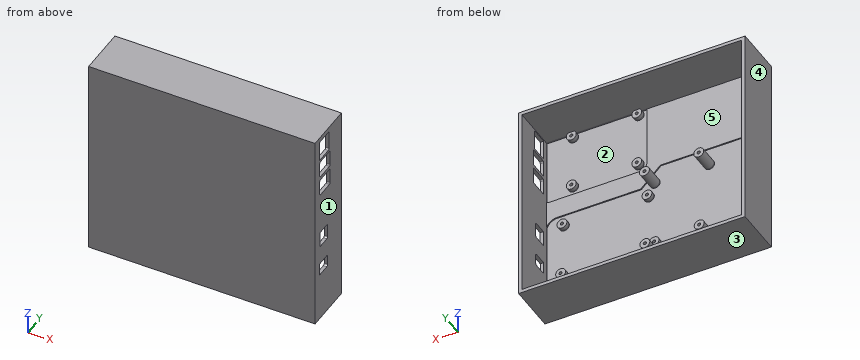
from build123d import *

# Parameters (mm, degrees)
SKETCH1_W           = 200.4
SKETCH1_H           = 180.383316975
SKETCH1_W_2         = 194.4
SKETCH1_H_2         = 174.383316975
BOSS_EXTRUDE1_DEPTH = 3
SKETCH1_3_W         = 200.4
SKETCH1_3_H         = 180.383316975
SKETCH1_3_W_2       = 194.4
SKETCH1_3_H_2       = 174.383316975
BOSS_EXTRUDE2_DEPTH = 40
SKETCH2_R           = 4.4
SKETCH2_R_2         = 1.4
BOSS_EXTRUDE3_DEPTH = 3
BOSS_EXTRUDE4_START = 3
SKETCH2_2_R         = 4.4
SKETCH2_2_R_2       = 1.4
BOSS_EXTRUDE4_DEPTH = 13.67
SKETCH3_R           = 4.4
CUT_EXTRUDE1_DEPTH  = 1
CUT_EXTRUDE2_DEPTH  = 5


with BuildPart() as part:
    # Sketch1 → Boss-Extrude1 (new body)
    with BuildSketch(Plane(origin=(0, -4, 0), x_dir=(-1, 0, 0), z_dir=(0, -1, 0))):
        with Locations((47.125, -25.608341513)):
            Rectangle(SKETCH1_W, SKETCH1_H)
        with Locations((47.125, -25.608341513)):
            Rectangle(SKETCH1_W_2, SKETCH1_H_2, mode=Mode.SUBTRACT)
        with Locations((47.125, -25.608341513)):
            Rectangle(SKETCH1_W_2, SKETCH1_H_2)
    extrude(amount=BOSS_EXTRUDE1_DEPTH)

    # Sketch1<3> → Boss-Extrude2 (add)
    with BuildSketch(Plane(origin=(0, -4, 0), x_dir=(-1, 0, 0), z_dir=(0, -1, 0))):
        with Locations((47.125, -25.608341513)):
            Rectangle(SKETCH1_3_W, SKETCH1_3_H)
        with Locations((47.125, -25.608341513)):
            Rectangle(SKETCH1_3_W_2, SKETCH1_3_H_2, mode=Mode.SUBTRACT)
    extrude(amount=-BOSS_EXTRUDE2_DEPTH)

    # Sketch2 → Boss-Extrude3 (add)
    with BuildSketch(Plane(origin=(0, -4, 0), x_dir=(1, 0, 0), z_dir=(0, 1, 0))):
        with Locations(Location((-94.083642028, 35.599553337, 0), (0, 0, 90))):
            Circle(SKETCH2_R)
        with Locations(Location((-94.083642028, 35.599553337, 0), (0, 0, 270))):
            Circle(SKETCH2_R_2, mode=Mode.SUBTRACT)
        with Locations(Location((-45.977533902, 35.843746779, 0), (0, 0, 90))):
            Circle(SKETCH2_R)
        with Locations(Location((-45.977533902, 35.843746779, 0), (0, 0, 270))):
            Circle(SKETCH2_R_2, mode=Mode.SUBTRACT)
        with Locations(Location((-46.675, 24.55, 0), (0, 0, 90))):
            Circle(SKETCH2_R)
        with Locations(Location((-46.675, 24.55, 0), (0, 0, 270))):
            Circle(SKETCH2_R_2, mode=Mode.SUBTRACT)
        with Locations(Location((35.975, 24.55, 0), (0, 0, 90))):
            Circle(SKETCH2_R)
        with Locations(Location((35.975, 24.55, 0), (0, 0, 270))):
            Circle(SKETCH2_R_2, mode=Mode.SUBTRACT)
        with Locations(Location((-40.425, -24.5, 0), (0, 0, 90))):
            Circle(SKETCH2_R)
        with Locations(Location((-40.425, -24.5, 0), (0, 0, 270))):
            Circle(SKETCH2_R_2, mode=Mode.SUBTRACT)
        with Locations(Location((-93.717351865, -36.559608852, 0), (0, 0, 90))):
            Circle(SKETCH2_R)
        with Locations(Location((-93.717351865, -36.559608852, 0), (0, 0, 270))):
            Circle(SKETCH2_R_2, mode=Mode.SUBTRACT)
        with Locations(Location((-45.611243739, -36.31541541, 0), (0, 0, 90))):
            Circle(SKETCH2_R)
        with Locations(Location((-45.611243739, -36.31541541, 0), (0, 0, 270))):
            Circle(SKETCH2_R_2, mode=Mode.SUBTRACT)
        with Locations(Location((34.775, -24.5, 0), (0, 0, 90))):
            Circle(SKETCH2_R)
        with Locations(Location((34.775, -24.5, 0), (0, 0, 270))):
            Circle(SKETCH2_R_2, mode=Mode.SUBTRACT)
        with Locations(Location((-31.425, -60.3, 0), (0, 0, 90))):
            Circle(SKETCH2_R)
        with Locations(Location((-31.425, -60.3, 0), (0, 0, 270))):
            Circle(SKETCH2_R_2, mode=Mode.SUBTRACT)
        with Locations(Location((26.575, -60.3, 0), (0, 0, 90))):
            Circle(SKETCH2_R)
        with Locations(Location((26.575, -60.3, 0), (0, 0, 270))):
            Circle(SKETCH2_R_2, mode=Mode.SUBTRACT)
        with Locations((-31.425, -109.3)):
            Circle(SKETCH2_R)
        with Locations(Location((-31.425, -109.3, 0), (0, 0, 270))):
            Circle(SKETCH2_R_2, mode=Mode.SUBTRACT)
        with Locations((26.575, -109.3)):
            Circle(SKETCH2_R)
        with Locations(Location((26.575, -109.3, 0), (0, 0, 270))):
            Circle(SKETCH2_R_2, mode=Mode.SUBTRACT)
    extrude(amount=BOSS_EXTRUDE3_DEPTH)

    # Sketch2<2> → Boss-Extrude4 (add)
    with BuildSketch(Plane(origin=(0, -4, 0), x_dir=(1, 0, 0), z_dir=(0, 1, 0)).offset(BOSS_EXTRUDE4_START)):
        with Locations(Location((-93.717351865, -36.559608852, 0), (0, 0, 90))):
            Circle(SKETCH2_2_R)
        with Locations(Location((-93.717351865, -36.559608852, 0), (0, 0, 270))):
            Circle(SKETCH2_2_R_2, mode=Mode.SUBTRACT)
        with Locations(Location((-45.611243739, -36.31541541, 0), (0, 0, 90))):
            Circle(SKETCH2_2_R)
        with Locations(Location((-45.611243739, -36.31541541, 0), (0, 0, 270))):
            Circle(SKETCH2_2_R_2, mode=Mode.SUBTRACT)
        with Locations(Location((-45.977533902, 35.843746779, 0), (0, 0, 90))):
            Circle(SKETCH2_2_R)
        with Locations(Location((-45.977533902, 35.843746779, 0), (0, 0, 270))):
            Circle(SKETCH2_2_R_2, mode=Mode.SUBTRACT)
        with Locations(Location((-94.083642028, 35.599553337, 0), (0, 0, 90))):
            Circle(SKETCH2_2_R)
        with Locations(Location((-94.083642028, 35.599553337, 0), (0, 0, 270))):
            Circle(SKETCH2_2_R_2, mode=Mode.SUBTRACT)
    extrude(amount=BOSS_EXTRUDE4_DEPTH)

    # Sketch3 → Cut-Extrude1 (cut)
    with BuildSketch(Plane(origin=(0, -4, 0), x_dir=(1, 0, 0), z_dir=(0, 1, 0))):
        with BuildLine():
            ThreePointArc((-133.325, -42.184637589), (-130.587997755, -49.351043774), (-123.472052941, -52.216683025))
            Line((-123.472052941, -52.216683025), (-50.730015352, -52.216683025))
            Line((-50.730015352, -52.216683025), (-33.377368591, -35.013077971))
            Line((-33.377368591, -35.013077971), (40.937843176, -35.013077971))
            ThreePointArc((40.937843176, -35.013077971), (46.610387698, -33.142667164), (50.075, -28.277211426))
            Line((50.075, -28.277211426), (50.075, 27.447920543))
            ThreePointArc((50.075, 27.447920543), (46.449358415, 32.437948869), (40.534398357, 34.186922029))
            Line((40.534398357, 34.186922029), (-33.678452679, 34.186922029))
            Line((-33.678452679, 34.186922029), (-50.108918246, 50.583316975))
            Line((-50.108918246, 50.583316975), (-124.102104511, 50.583316975))
            ThreePointArc((-124.102104511, 50.583316975), (-130.528855148, 47.775760881), (-133.325, 41.344037245))
            Line((-133.325, 41.344037245), (-133.325, -42.184637589))
        make_face()
        with Locations(Location((-93.717351865, -36.559608852, 0), (0, 0, 270))):
            Circle(SKETCH3_R, mode=Mode.SUBTRACT)
        with Locations(Location((-45.611243739, -36.31541541, 0), (0, 0, 270))):
            Circle(SKETCH3_R, mode=Mode.SUBTRACT)
        with Locations(Location((-94.083642028, 35.599553337, 0), (0, 0, 270))):
            Circle(SKETCH3_R, mode=Mode.SUBTRACT)
        with Locations(Location((-40.425, -24.5, 0), (0, 0, 270))):
            Circle(SKETCH3_R, mode=Mode.SUBTRACT)
        with Locations(Location((34.775, -24.5, 0), (0, 0, 270))):
            Circle(SKETCH3_R, mode=Mode.SUBTRACT)
        with Locations(Location((-46.675, 24.55, 0), (0, 0, 270))):
            Circle(SKETCH3_R, mode=Mode.SUBTRACT)
        with Locations(Location((-45.977533902, 35.843746779, 0), (0, 0, 270))):
            Circle(SKETCH3_R, mode=Mode.SUBTRACT)
        with Locations(Location((35.975, 24.55, 0), (0, 0, 270))):
            Circle(SKETCH3_R, mode=Mode.SUBTRACT)
        with BuildLine():
            Line((50.075, -112.8), (50.075, -53.47544468))
            ThreePointArc((50.075, -53.47544468), (48.612548822, -52.970948556), (47.075, -52.8))
            Line((47.075, -52.8), (-31.925, -52.8))
            ThreePointArc((-31.925, -52.8), (-36.874747468, -54.850252532), (-38.925, -59.8))
            Line((-38.925, -59.8), (-38.925, -109.8))
            ThreePointArc((-38.925, -109.8), (-38.754051444, -111.337548822), (-38.24955532, -112.8))
            Line((-38.24955532, -112.8), (-34.091458325, -112.8))
            ThreePointArc((-34.091458325, -112.8), (-31.425, -104.9), (-28.758541675, -112.8))
            Line((-28.758541675, -112.8), (23.908541675, -112.8))
            ThreePointArc((23.908541675, -112.8), (26.575, -104.9), (29.241458325, -112.8))
            Line((29.241458325, -112.8), (50.075, -112.8))
        make_face()
        with Locations(Location((-31.425, -60.3, 0), (0, 0, 270))):
            Circle(SKETCH3_R, mode=Mode.SUBTRACT)
        with Locations(Location((26.575, -60.3, 0), (0, 0, 270))):
            Circle(SKETCH3_R, mode=Mode.SUBTRACT)
    extrude(amount=-CUT_EXTRUDE1_DEPTH, mode=Mode.SUBTRACT)

    # Sketch4 → Cut-Extrude2 (cut)
    with BuildSketch(Plane(origin=(53.075, 0, 0), x_dir=(0, 0, -1), z_dir=(1, 0, 0))):
        with BuildLine():
            Line((9.9, 0.63), (20.9, 0.63))
            Line((20.9, 0.63), (20.9, 12.13))
            ThreePointArc((20.9, 12.13), (20.460660172, 13.190660172), (19.4, 13.63))
            Line((19.4, 13.63), (11.4, 13.63))
            ThreePointArc((11.4, 13.63), (10.339339828, 13.190660172), (9.9, 12.13))
            Line((9.9, 12.13), (9.9, 0.63))
        make_face()
        with BuildLine():
            Line((-8.32, 13.68), (-19.44, 13.68))
            ThreePointArc((-19.44, 13.68), (-20.472375901, 13.252375901), (-20.9, 12.22))
            Line((-20.9, 12.22), (-20.9, 12.12))
            Line((-20.9, 12.12), (-20.9, 2.47))
            Line((-20.9, 2.47), (-20.9, 1.06))
            Line((-20.9, 1.06), (-6.86, 1.06))
            Line((-6.86, 1.06), (-6.86, 2.47))
            Line((-6.86, 2.47), (-6.86, 12.12))
            Line((-6.86, 12.12), (-6.86, 12.22))
            ThreePointArc((-6.86, 12.22), (-7.287624099, 13.252375901), (-8.32, 13.68))
        make_face()
        with BuildLine():
            Line((-71.3, 17.63), (-60.3, 17.63))
            Line((-60.3, 17.63), (-59.55, 17.63))
            ThreePointArc((-59.55, 17.63), (-58.990983006, 17.498033989), (-58.55, 17.13))
            ThreePointArc((-58.55, 17.13), (-58.364145877, 16.775284708), (-58.3, 16.38))
            Line((-58.3, 16.38), (-58.3, 15.13))
            Line((-58.3, 15.13), (-58.3, 3.13))
            Line((-58.3, 3.13), (-58.3, 1.88))
            ThreePointArc((-58.3, 1.88), (-58.364145877, 1.484715292), (-58.55, 1.13))
            ThreePointArc((-58.55, 1.13), (-58.990983006, 0.761966011), (-59.55, 0.63))
            Line((-59.55, 0.63), (-60.3, 0.63))
            Line((-60.3, 0.63), (-71.3, 0.63))
            Line((-71.3, 0.63), (-72.05, 0.63))
            ThreePointArc((-72.05, 0.63), (-72.609016994, 0.761966011), (-73.05, 1.13))
            ThreePointArc((-73.05, 1.13), (-73.235854123, 1.484715292), (-73.3, 1.88))
            Line((-73.3, 1.88), (-73.3, 3.13))
            Line((-73.3, 3.13), (-73.3, 15.13))
            Line((-73.3, 15.13), (-73.3, 16.38))
            ThreePointArc((-73.3, 16.38), (-73.235854123, 16.775284708), (-73.05, 17.13))
            ThreePointArc((-73.05, 17.13), (-72.609016994, 17.498033989), (-72.05, 17.63))
            Line((-72.05, 17.63), (-71.3, 17.63))
        make_face()
        with BuildLine():
            Line((-90.05, 0.63), (-89.3, 0.63))
            Line((-89.3, 0.63), (-78.3, 0.63))
            Line((-78.3, 0.63), (-77.55, 0.63))
            ThreePointArc((-77.55, 0.63), (-76.990983006, 0.761966011), (-76.55, 1.13))
            ThreePointArc((-76.55, 1.13), (-76.364145877, 1.484715292), (-76.3, 1.88))
            Line((-76.3, 1.88), (-76.3, 3.13))
            Line((-76.3, 3.13), (-76.3, 15.13))
            Line((-76.3, 15.13), (-76.3, 16.38))
            ThreePointArc((-76.3, 16.38), (-76.364145877, 16.775284708), (-76.55, 17.13))
            ThreePointArc((-76.55, 17.13), (-76.990983006, 17.498033989), (-77.55, 17.63))
            Line((-77.55, 17.63), (-78.3, 17.63))
            Line((-78.3, 17.63), (-89.3, 17.63))
            Line((-89.3, 17.63), (-90.05, 17.63))
            ThreePointArc((-90.05, 17.63), (-90.609016994, 17.498033989), (-91.05, 17.13))
            ThreePointArc((-91.05, 17.13), (-91.235854123, 16.775284708), (-91.3, 16.38))
            Line((-91.3, 16.38), (-91.3, 15.13))
            Line((-91.3, 15.13), (-91.3, 3.13))
            Line((-91.3, 3.13), (-91.3, 1.88))
            ThreePointArc((-91.3, 1.88), (-91.235854123, 1.484715292), (-91.05, 1.13))
            ThreePointArc((-91.05, 1.13), (-90.609016994, 0.761966011), (-90.05, 0.63))
        make_face()
        with BuildLine():
            Line((-93.55, 14.73), (-93.55, 1.63))
            Line((-93.55, 1.63), (-93.55, 0.63))
            Line((-93.55, 0.63), (-100.55, 0.63))
            Line((-100.55, 0.63), (-104.55, 0.63))
            Line((-104.55, 0.63), (-111.55, 0.63))
            Line((-111.55, 0.63), (-111.55, 1.63))
            Line((-111.55, 1.63), (-111.55, 14.73))
            ThreePointArc((-111.55, 14.73), (-111.198528137, 15.578528137), (-110.35, 15.93))
            Line((-110.35, 15.93), (-94.75, 15.93))
            ThreePointArc((-94.75, 15.93), (-93.901471863, 15.578528137), (-93.55, 14.73))
        make_face()
    extrude(amount=-CUT_EXTRUDE2_DEPTH, mode=Mode.SUBTRACT)


solid = part.part
Source: CAD feature listing. Evaluate the final solid. Frame: model axes, mm. Face numbers are marked on the shaded views. A direction names the side the tool comes from. Round coordinates to 2 decimals unless told otherwise and drop trailing zeros. Order: outer loops, then holes, each group sorted by start corner. A loop starts at its lowest first (then second) coordinate and runs counter-clockwise, first axis right, second up. Notation, with made-up numbers: (-37.5, 14.5) -> (-17.5, 14.5) arc R26 ccw to (-17.5, 32.5) -> close; hole circle Ø2 at (12.5, 54.25). An arc over 180 degrees is marked (long way). Answer as CSV lines item,"result".
Item 1: Section A-A, the plane z = 85. Return loops of the section in (x, y) (3 decimals).
A:
outline,"(-147.325, -7) -> (53.075, -7) -> (53.075, 0.63) -> (50.075, 0.63) -> (50.075, -5) -> (-38.925, -5) -> (-38.925, -4) -> (-144.325, -4) -> (-144.325, 36) -> (-147.325, 36) -> close; (50.075, 17.63) -> (53.075, 17.63) -> (53.075, 36) -> (50.075, 36) -> close"
Item 2: Section D-D, the plane x = -117. Return loops of the section in (y, z), plus the area to 3 significant figures.
A:
outline,"(-7, -64.58) -> (36, -64.58) -> (36, -61.58) -> (-4, -61.58) -> (-4, -50.58) -> (-5, -50.58) -> (-5, 52.22) -> (-4, 52.22) -> (-4, 112.8) -> (36, 112.8) -> (36, 115.8) -> (-7, 115.8) -> close"
area,"678 mm²"
Item 3: Pin query (flat end, axial travel): pin 1 Ø8 at (x, z) = (-37, -5.5) entering from +Y; pin 2 Ø4.5 at (x, z) = (-93.5, -33.5) entering from +Y; pin 3 Ø9.5 at (x, z) = (-42.5, 24.5) entering from +Y. Return the tip coordinate at first contact, or that it passes through.
A:
pin 1,"y = -5"
pin 2,"y = 12.67"
pin 3,"y = -1"
Item 4: Section B-B, the plane x = -7. Return loops of the section in (y, z), plus the area to 3 significant figures.
A:
outline,"(-7, -64.58) -> (36, -64.58) -> (36, -61.58) -> (-4, -61.58) -> (-4, -34.19) -> (-5, -34.19) -> (-5, 35.01) -> (-4, 35.01) -> (-4, 52.8) -> (-5, 52.8) -> (-5, 112.8) -> (36, 112.8) -> (36, 115.8) -> (-7, 115.8) -> close"
area,"652 mm²"
Item 5: Pull-direction query (Z, two-part tool) for the marked faces 1, 2 and 3; classes: pulls with the +Z half, pulls with the -Z half, needs draft (parallel to the pull), parting line crosses it, or undercut.
A:
face 1,"needs draft"
face 2,"undercut"
face 3,"pulls with the -Z half"
Item 6: Line query: L1, parallel to X at y = -1.65, z = 24.5 (3 decimals); L2, parallel to X at y = 9, z = 53.5 (3 decimals); L3, parallel to Z at x = -118.5, y = 3. Output: solid intervals per line, ascending.
A:
L1,"-147.325 to -144.325, -44.825 to -41.825, -39.025 to -36.025, 30.375 to 33.375, 36.175 to 39.175, 50.075 to 53.075"
L2,"-147.325 to -144.325, 50.075 to 53.075"
L3,"-64.58 to -61.58, 112.8 to 115.8"
Item 7: Reachability of the marked faces 4 and 5 from +Z, -Z, +X, -X, +Y, -Y: full face, straight path, thin tool, end or side. Return the list, or none.
A:
face 4,"+Z, -Z, -X, +Y, -Y"
face 5,"+Y"
Item 8: Section C-C, the plane y = 8. Count the separate pieces of the cut face and the enclosed holes in it, plus the area to 3 significant figures.
A:
separate pieces,"9"
enclosed holes,"4"
area,"2,250 mm²"
